from build123d import *

# Parameters (mm, degrees)
SKETCH1_W           = 20
SKETCH1_H           = 20
BOSS_EXTRUDE2_DEPTH = 30
SKETCH2_R           = 5
BOSS_EXTRUDE3_DEPTH = 10
CUT_EXTRUDE2_DEPTH  = 20
SKETCH5_W           = 20
SKETCH5_H           = 30
BOSS_EXTRUDE4_DEPTH = 30
CUT_EXTRUDE3_DEPTH  = 20
SKETCH7_W           = 20
SKETCH7_H           = 40
BOSS_EXTRUDE5_DEPTH = 10
SKETCH8_W           = 20
SKETCH8_H           = 10
BOSS_EXTRUDE6_DEPTH = 15
CUT_EXTRUDE4_DEPTH  = 20
SKETCH10_R          = 2.481643059
BOSS_EXTRUDE7_DEPTH = 10


with BuildPart() as part:
    # Sketch1 → Boss-Extrude2 (new body)
    with BuildSketch(Plane(origin=(0, 0, 0), x_dir=(1, 0, 0), z_dir=(0, 1, 0))):
        with Locations((1.888111888, -1.538461538)):
            Rectangle(SKETCH1_W, SKETCH1_H)
    extrude(amount=BOSS_EXTRUDE2_DEPTH)

    # Sketch2 → Boss-Extrude3 (add)
    with BuildSketch(Plane(origin=(11.888111888, 0, 0), x_dir=(0, 0, -1), z_dir=(1, 0, 0))):
        with Locations(Location((-1.538461538, 10, 0), (0, 0, 180))):
            Circle(SKETCH2_R)
    boss_extrude3 = extrude(amount=BOSS_EXTRUDE3_DEPTH)

    # Mirror1: Boss-Extrude3 across plane
    add(boss_extrude3.mirror(Plane(origin=(1.888111888, 0, 0), x_dir=(0, 0, 1), z_dir=(1, 0, 0))))

    # Sketch3 → Cut-Extrude2 (cut)
    with BuildSketch(Plane(origin=(11.888111888, 0, 0), x_dir=(0, 0, -1), z_dir=(1, 0, 0))):
        Polygon((-11.538461538, 0), (-3.87574726, 30), (-11.538461538, 30), align=None)
    extrude(amount=-CUT_EXTRUDE2_DEPTH, mode=Mode.SUBTRACT)

    # Sketch5 → Boss-Extrude4 (add)
    with BuildSketch(Plane(origin=(0, 30, 0), x_dir=(1, 0, 0), z_dir=(0, 1, 0))):
        with Locations((1.888111888, -6.538461538)):
            Rectangle(SKETCH5_W, SKETCH5_H)
    extrude(amount=BOSS_EXTRUDE4_DEPTH)

    # Sketch6 → Cut-Extrude3 (cut)
    with BuildSketch(Plane(origin=(11.888111888, 0, 0), x_dir=(0, 0, -1), z_dir=(1, 0, 0))):
        Polygon((-3.87574726, 30), (-21.538461538, 60), (-21.538461538, 30), align=None)
        Polygon((8.461538462, 30), (8.461538462, 60), (-11.538461538, 60), align=None)
    extrude(amount=-CUT_EXTRUDE3_DEPTH, mode=Mode.SUBTRACT)

    # Sketch7 → Boss-Extrude5 (add)
    with BuildSketch(Plane(origin=(0, 60, 0), x_dir=(1, 0, 0), z_dir=(0, 1, 0))):
        with Locations((1.888111888, -31.538461538)):
            Rectangle(SKETCH7_W, SKETCH7_H)
    extrude(amount=BOSS_EXTRUDE5_DEPTH)

    # Sketch8 → Boss-Extrude6 (add)
    with BuildSketch(Plane(origin=(0, 70, 0), x_dir=(1, 0, 0), z_dir=(0, 1, 0))):
        with Locations((1.888111888, -46.538461538)):
            Rectangle(SKETCH8_W, SKETCH8_H)
    extrude(amount=BOSS_EXTRUDE6_DEPTH)

    # Sketch9 → Cut-Extrude4 (cut)
    with BuildSketch(Plane(origin=(11.888111888, 0, 0), x_dir=(0, 0, -1), z_dir=(1, 0, 0))):
        Polygon((-51.538461538, 70), (-47.598538903, 85), (-51.538461538, 85), align=None)
    extrude(amount=-CUT_EXTRUDE4_DEPTH, mode=Mode.SUBTRACT)

    # Sketch10 → Boss-Extrude7 (add)
    with BuildSketch(Plane(origin=(0, 85, 0), x_dir=(1, 0, 0), z_dir=(0, 1, 0))):
        with Locations(Location((1.888111888, -44.588461538, 0), (0, 0, 270))):
            Circle(SKETCH10_R)
    extrude(amount=BOSS_EXTRUDE7_DEPTH)


solid = part.part
Geometry check sheet. Reference: the model listing, model coordinates, mm. A direction names the side the tool comes from. Give positions to 0.01 mm unless a question says otherwise; leave off trailing zeros. Order: outer loops, then holes, each group sorted by start corner. A loop starts at its lowest first (then second) coordinate and runs counter-clockwise, first axis right, second up. Notation, with made-up numbers: (45, 84.25) - (49, 84.25) arc R12 cw to (49, 97.25) - close; hole circle Ø1 at (19.25, -36). An arc over 180 degrees is marked (long way). Answer as a JSON object with one key per item and string values.
(1) Tool access check on faces 4 (the flat face through (2, 60, 36)), 5 (the flat face through (2.03, 14.79, 7.76)), 6 (the flat face through (2, 65, 11.538)). Record the directions out of +Z, -Z, +X, -X, +Y, -Y that give a thin tool (end or side, any length) a straight path to the whole face; none if there is none.
Report:
{"face 4": "+Z, +X, -X, -Y", "face 5": "+Z, +X, -X", "face 6": "-Z, +X, -X, +Y"}
(2) Cross-section at A-A (z = 5.5). Record the cut outline in (x, y), then the cut area to 3 significant figures.
Report:
{"outline": "(-18.11, 6.95) - (-8.11, 6.95) - (-8.11, 0) - (11.89, 0) - (11.89, 6.95) - (21.89, 6.95) - (21.89, 13.05) - (11.89, 13.05) - (11.89, 23.64) - (-8.11, 23.64) - (-8.11, 13.05) - (-18.11, 13.05) - close; (-8.11, 32.76) - (11.89, 32.76) - (11.89, 50.94) - (-8.11, 50.94) - close", "area": "959 mm^2"}
(3) Draft check along Y on faces 1 (the flat face through (2, 95, 45)), 2 (the flat face through (2, 77, 41.538)), 3 (the flat face through (2.028, 44.79, 12.583)). Enter one of: released by +Y, released by -Y, zero draft, split by the parting line, or undercut.
Report:
{"face 1": "released by +Y", "face 2": "zero draft", "face 3": "undercut"}
(4) Cross-section at D-D (z = 24). Record the cut outline in (x, y), then the cut area to 3 significant figures.
Report:
{"outline": "(-8.11, 60) - (11.89, 60) - (11.89, 70) - (-8.11, 70) - close", "area": "200 mm^2"}
(5) Depth check by flat-ended pin: pin 1 Ø12 at (x, y) = (-2.5, 74) entering from -Z; pin 2 Ø10 at (x, y) = (5.5, 48.5) entering from -Z; pin 3 Ø12 at (x, y) = (0.5, 51.5) entering from -Z; pin 4 Ø5 at (x, z) = (6, 45) entering from +Y. Enter the tip coordinate at first touch or a pass-through.
Report:
{"pin 1": "z = 11.54", "pin 2": "z = 0.54", "pin 3": "z = 1.87", "pin 4": "y = 95"}
(6) Cross-section at C-C (y = 10). Record the cut outline in (x, z).
Report:
{"outline": "(-18.11, -3.46) - (-8.11, -3.46) - (-8.11, -8.46) - (11.89, -8.46) - (11.89, -3.46) - (21.89, -3.46) - (21.89, 6.54) - (11.89, 6.54) - (11.89, 8.98) - (-8.11, 8.98) - (-8.11, 6.54) - (-18.11, 6.54) - close"}
(7) Cross-section at B-B (x = 6.5). Record the cut outline in (y, z).
Report:
{"outline": "(0, -8.46) - (30, -8.46) - (60, 11.54) - (70, 11.54) - (70, 41.54) - (85, 41.54) - (85, 47.6) - (70, 51.54) - (60, 51.54) - (60, 21.54) - (30, 3.88) - (0, 11.54) - close"}
(8) Material ranges on line 1 (Z direction, x = 2.5, y = 66.5); line 2 (X direction, y = 65, z = 16); line 3 (Y direction, x = -6, z = 27), recorded low to high.
Report:
{"line 1": "11.54 to 51.54", "line 2": "-8.11 to 11.89", "line 3": "60 to 70"}
